Verification items for the finished model (mm, model axes). Round coordinates to 2 decimals unless told otherwise and drop trailing zeros. Write each loop counter-clockwise with the first axis right and the second up, starting at its lowest first coordinate (ties: lowest second). Pieces come first, ordered by that corner, then holes. Notation, with made-up numbers: M -5,70 L 54,70 A18 cw 54,83 Z; hole C 16,75 d11. An arc over 180 degrees is marked long. Answer in a Markdown table with one row per item. Add a question column.
1. Sectioned sample at A-A on y = 6.25. Record the cut outline in (x, z).
2. Material ranges on probe 1 along Z at (x, y) = (0, 3); probe 2 along Y at (x, z) = (-6, -12.5); probe 3 along Z at (x, y) = (1, 0.5), recorded low to high.
3. Draft check along X on faces 1 (the flat face through (0, 5, -2.05)), 2 (the cylindrical face through (-7.086, 2.218, 17.089)), 3 (the flat face through (-4, 10, 0)). Enter one of: pulls with the +X half, pulls with the -X half, needs draft (parallel to the pull), parting line crosses it, or undercut.
4. Go/stop test with flat-tipped pins: pin 1 Ø4 at (x, y) = (-3, 8.5) entering from -Z; pin 2 Ø6 at (x, z) = (-8, -1.5) entering from -Y; pin 3 Ø5 at (x, y) = (7, 6) entering from -Z; pin 4 Ø1.5 at (y, z) = (3.5, -2) entering from +X. Record where each tip stops, or that it passes through.
```python
from build123d import *

# Parameters (mm, degrees)
SKETCH1_R                                 = 18.5
BOSS_EXTRUDE1_DEPTH                       = 10
SKETCH2_R                                 = 0.5
CUT_EXTRUDE1_REACH                        = 30.009
CUT_EXTRUDE2_REACH                        = 30.009
CUT_EXTRUDE2_END_MAJOR_RADIUS             = 18.5
CUT_EXTRUDE2_END_MINOR_RADIUS             = 0.5
SKETCH4_R                                 = 0.5
CUT_EXTRUDE2_DIRECTION_2_REACH            = 30.009
CUT_EXTRUDE2_DIRECTION_2_END_MAJOR_RADIUS = 18.5
CUT_EXTRUDE2_DIRECTION_2_END_MINOR_RADIUS = 0.5


with BuildPart() as part:
    # Sketch1 → Boss-Extrude1 (new body)
    with BuildSketch(Plane(origin=(0, 0, 0), x_dir=(1, 0, 0), z_dir=(0, 1, 0))):
        with Locations(Location((0, 0, 0), (0, 0, 270))):
            Circle(SKETCH1_R)
    extrude(amount=BOSS_EXTRUDE1_DEPTH)

    # Sketch2 → Cut-Revolve1 (revolve, cut)
    with BuildSketch(Plane.XY, mode=Mode.PRIVATE) as cut_revolve1_sk:
        with Locations((-18.5, 5)):
            Circle(SKETCH2_R)
    revolve(cut_revolve1_sk.sketch.rotate(Axis((0, 22.422972825, 0), (0, -1, 0)), 270), axis=Axis((0, 22.422972825, 0), (0, -1, 0)), mode=Mode.SUBTRACT)

    # Sketch3 → Cut-Extrude1 (cut, up to next)
    with BuildSketch(Plane(origin=(0, 10, 0), x_dir=(1, 0, 0), z_dir=(0, 1, 0)), mode=Mode.PRIVATE) as cut_extrude1_sk1:
        with BuildLine():
            Line((1.516575089, 2.05), (-1.516575089, 2.05))
            ThreePointArc((-1.516575089, 2.05), (-1.147874889, -2.277033868), (2.55, 0))
            ThreePointArc((2.55, 0), (2.277033868, 1.147874889), (1.516575089, 2.05))
        make_face()
    cut_extrude1_tool1 = extrude(cut_extrude1_sk1.sketch, amount=-CUT_EXTRUDE1_REACH, mode=Mode.PRIVATE) & part.part
    add(cut_extrude1_tool1.solids().sort_by_distance((0, 10, 0.119895))[0], mode=Mode.SUBTRACT)

    # Cut-Extrude2: up to this torus (the profile starts outside it)
    cut_extrude2_end = Plane(origin=(0, 5, 0), z_dir=(0, 1, 0)) * Torus(CUT_EXTRUDE2_END_MAJOR_RADIUS, CUT_EXTRUDE2_END_MINOR_RADIUS, mode=Mode.PRIVATE)
    # Sketch4 → Cut-Extrude2 (cut, up to the surface)
    with BuildSketch(Plane.XY, mode=Mode.PRIVATE) as cut_extrude2_sk1:
        with Locations(Location((-6, 5, 0), (0, 0, 90))):
            Circle(SKETCH4_R)
    cut_extrude2_tool1 = extrude(cut_extrude2_sk1.sketch, amount=-CUT_EXTRUDE2_REACH, mode=Mode.PRIVATE) - cut_extrude2_end
    add(cut_extrude2_tool1.solids().sort_by_distance((-6, 5, 0))[0], mode=Mode.SUBTRACT)

    # Cut-Extrude2 direction 2: up to this torus (the profile starts outside it)
    cut_extrude2_direction_2_end = Plane(origin=(0, 5, 0), z_dir=(0, 1, 0)) * Torus(CUT_EXTRUDE2_DIRECTION_2_END_MAJOR_RADIUS, CUT_EXTRUDE2_DIRECTION_2_END_MINOR_RADIUS, mode=Mode.PRIVATE)
    # Sketch4 → Cut-Extrude2 direction 2 (cut, up to the surface)
    with BuildSketch(Plane.XY, mode=Mode.PRIVATE) as cut_extrude2_direction_2_sk1:
        with Locations(Location((-6, 5, 0), (0, 0, 90))):
            Circle(SKETCH4_R)
    cut_extrude2_direction_2_tool1 = extrude(cut_extrude2_direction_2_sk1.sketch, amount=CUT_EXTRUDE2_DIRECTION_2_REACH, mode=Mode.PRIVATE) - cut_extrude2_direction_2_end
    add(cut_extrude2_direction_2_tool1.solids().sort_by_distance((-6, 5, 0))[0], mode=Mode.SUBTRACT)


solid = part.part
```
Geometry check:
| question | item | result |
|---|---|---|
| 1 | outline | C 0,0 d37; hole M -1.52,-2.05 L 1.52,-2.05 A2.55 ccw long Z |
| 2 | probe 1 | z = -18.5 to -2.05, 2.55 to 18.5 |
| 2 | probe 2 | y = 0 to 4.5, 5.5 to 10 |
| 2 | probe 3 | z = -18.47 to -2.05, 2.35 to 18.47 |
| 3 | face 1 | undercut |
| 3 | face 2 | parting line crosses it |
| 3 | face 3 | needs draft |
| 4 | pin 1 | stops at z = -18.47 |
| 4 | pin 2 | stops at y = 0 |
| 4 | pin 3 | stops at z = -17.94 |
| 4 | pin 4 | stops at x = 18.46 |
